Verification items for the finished model (mm, model axes). Give positions to 0.01 mm unless a question says otherwise; leave off trailing zeros. Order: outer loops, then holes, each group sorted by start corner. A loop starts at its lowest first (then second) coordinate and runs counter-clockwise, first axis right, second up.
from build123d import *

# Parameters (mm, degrees)
F0_R     = 5.05
F0_W     = 2.5
F0_H     = 10
F1_DEPTH = 10
F2_R     = 4
F3_R     = 1


# Not quite as in the source:
# - a feature names something its author has since deleted; it is built from what else it names


with BuildPart() as f1:
    # F0 (on Front) → F1 (new body)
    with BuildSketch(Plane.XZ):
        with BuildLine():
            Line((-79.75, 79.75), (-79.75, -79.75))
            Line((-79.75, -79.75), (-2.5, -79.75))
            Line((-2.5, -79.75), (-2.5, -69.75))
            Line((-2.5, -69.75), (-2.5, -60.6985378737))
            ThreePointArc((-2.5, -60.6985378737), (-6.0183598459, -60.4511525512), (-9.5164331553, -60))
            ThreePointArc((-9.5164331553, -60), (-60.6476127119, 3.5255598628), (-2.5, 60.6985378737))
            Line((-2.5, 60.6985378737), (-2.5, 79.75))
            Line((-2.5, 79.75), (-79.75, 79.75))
        make_face()
        with Locations((-60, -60)):
            Circle(F0_R, mode=Mode.SUBTRACT)
        with BuildLine():
            Line((2.5, -69.75), (2.5, -79.75))
            Line((2.5, -79.75), (79.75, -79.75))
            Line((79.75, -79.75), (79.75, 79.75))
            Line((79.75, 79.75), (2.5, 79.75))
            Line((2.5, 79.75), (2.5, 60.6985378737))
            ThreePointArc((2.5, 60.6985378737), (43.8317094123, 42.0635679656), (60.75, 0))
            ThreePointArc((60.75, 0), (46.198949199, -39.448949199), (9.5164331553, -60))
            ThreePointArc((9.5164331553, -60), (6.0183598459, -60.4511525512), (2.5, -60.6985378737))
            Line((2.5, -60.6985378737), (2.5, -69.75))
        make_face()
        with BuildLine():
            ThreePointArc((65.05, -60), (60, -65.05), (54.95, -60))
            ThreePointArc((54.95, -60), (60, -54.95), (65.05, -60))
        make_face(mode=Mode.SUBTRACT)
        with Locations((-1.25, -74.75)):
            Rectangle(F0_W, F0_H)
        with Locations((1.25, -74.75)):
            Rectangle(F0_W, F0_H)
    extrude(amount=F1_DEPTH)

    # F2
    f2_edges = [f1.edges().sort_by_distance(p)[0] for p in [
        (79.75, -5, 79.75),
        (-79.75, -5, 79.75),
        (-79.75, -5, -79.75),
        (79.75, -5, -79.75),
        (-2.5, -5, 60.698538),
        (-2.5, -5, 79.75),
        (2.5, -5, 79.75),
        (2.5, -5, 60.698538),
        (2.5, -5, -60.698538),
        (-2.5, -5, -60.698538),
    ]]
    fillet(f2_edges, radius=F2_R)

    # F3
    f3_edges = [f1.edges().sort_by_distance(p)[0] for p in [
        (-2.5, -5, -69.75),
        (2.5, -5, -69.75),
    ]]
    fillet(f3_edges, radius=F3_R)


solid = f1.part
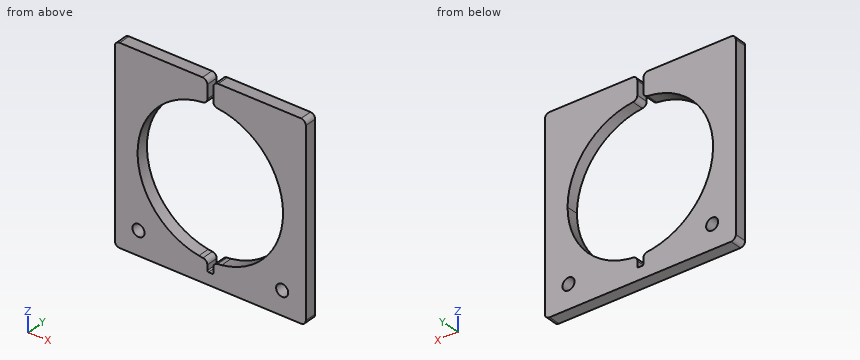
(1) Section check C-C, the plane z = 35. Enter the section's corners in (x, y).
Solved:
outline: (-79.75, -10) - (-49.65, -10) - (-49.65, 0) - (-79.75, 0) - close; (49.65, -10) - (79.75, -10) - (79.75, 0) - (49.65, 0) - close
(2) Section check B-B, the plane x = 29.5. Enter the section's corners in (y, z), then the cut area to 3 significant figures.
Solved:
outline: (-10, -79.75) - (0, -79.75) - (0, -53.11) - (-10, -53.11) - close; (-10, 53.11) - (0, 53.11) - (0, 79.75) - (-10, 79.75) - close
area: 533 mm2
(3) Section check A-A, the plane y = -3.75. Enter the section's corners in (x, z).
Solved:
outline: (-79.75, -75.75) arc R4 ccw to (-75.75, -79.75) - (75.75, -79.75) arc R4 ccw to (79.75, -75.75) - (79.75, 75.75) arc R4 ccw to (75.75, 79.75) - (6.5, 79.75) arc R4 ccw to (2.5, 75.75) - (2.5, 64.42) arc R4 ccw to (6.1, 60.44) arc R60.75 cw to (6.1, -60.44) arc R4 ccw to (2.5, -64.42) - (2.5, -68.75) arc R1 cw to (1.5, -69.75) - (-1.5, -69.75) arc R1 cw to (-2.5, -68.75) - (-2.5, -64.42) arc R4 ccw to (-6.1, -60.44) arc R60.75 cw to (-6.1, 60.44) arc R4 ccw to (-2.5, 64.42) - (-2.5, 75.75) arc R4 ccw to (-6.5, 79.75) - (-75.75, 79.75) arc R4 ccw to (-79.75, 75.75) - close; hole circle Ø10.1 at (-60, -60); hole circle Ø10.1 at (60, -60)
(4) Go/stop test with flat-tipped pins: pin 1 (3.5 mm diameter, centred on x = 0.5, y = -7, fed in from +Z); pin 2 (9 mm diameter, centred on x = -60, z = -60, fed in from +Y). Record where each tip stops, or that it passes through.
Solved:
pin 1: stops at z = -69.41
pin 2: passes through
(5) Scan lines: line 1 (X direction, y = -3.5, z = 70); line 2 (Z direction, x = 15.5, y = -7.5); line 3 (Z direction, x = 9, y = -0.75). Record each from-to range of solid material in increasing order.
Solved:
line 1: x = -79.75 to -2.5, 2.5 to 79.75
line 2: z = -79.75 to -58.74, 58.74 to 79.75
line 3: z = -79.75 to -60.08, 60.08 to 79.75
